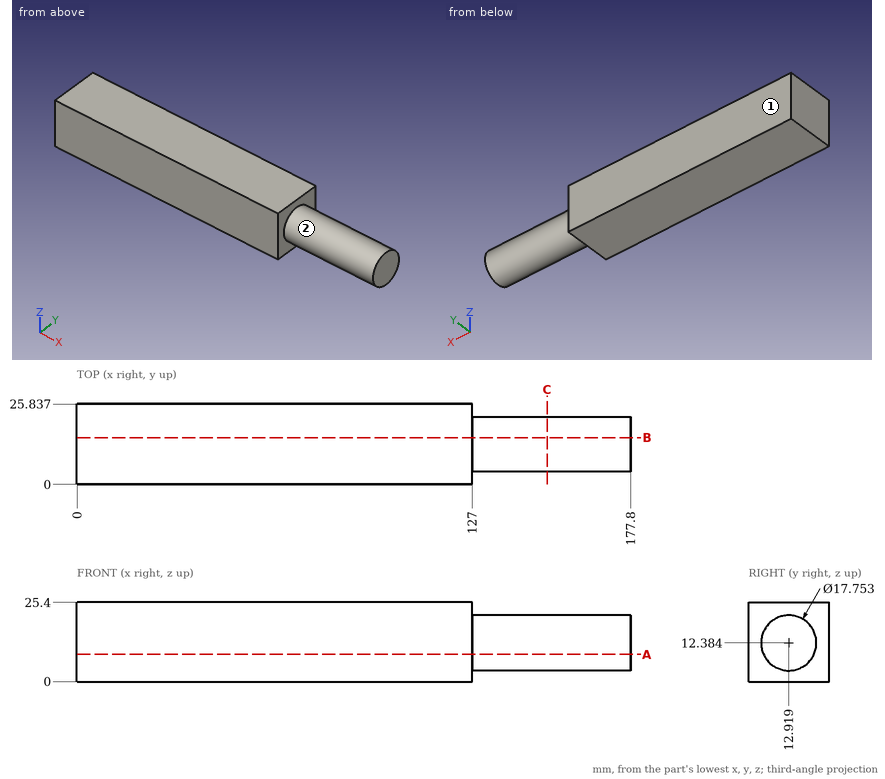
Here's the drawing with two shaded views (mm, measured from the low corner). I have some questions. A direction names the side the tool comes from. Coordinates: 2 decimals unless noted, no trailing zeros. Write each loop counter-clockwise with the first axis right and the second up, starting at its lowest first coordinate (ties: lowest second). Pieces come first, ordered by that corner, then holes. Notation, with made-up numbers: M 34.5,55 L 57.5,55 A6 ccw 57.5,66 Z; hole C 54.5,-13.75 d7. An arc over 180 degrees is marked long. Answer as CSV lines item,"result". Start each with the question number.
1) I want a section at A-A, the plane z = 8.75. Please give me the cut outline in (x, y), and give its area (3 significant figures).
2) I want a section at B-B, the plane y = 15. Please give me the cut outline in (x, z) (1 decimal).
3) For the marked faces 1 and 2, which set-ups out of +Z, -Z, +X, -X, +Y, -Y let a thin tool reach every point of the face, with its end or its side?
4) Please list where these lines run through material, in increasing order: line 1 (X direction, y = 5.5, z = 21.75); line 2 (Y direction, x = 142, z = 5) (1 decimal); line 3 (Z direction, x = 133, y = 19). Write a range as from..to.
5) I want a section at C-C, the plane x = 151. Please give me the cut outline in (y, z) (1 decimal).
6) For P1, Ø6, axis at x = 153.5, y = 7, coming from the -Z side, with a flat end and sliding along its axis, tell me the tip position at first contact or that it passes through.
Data:
1,outline,"M 0,0 L 127,0 L 127,4.82 L 177.8,4.82 L 177.8,21.02 L 127,21.02 L 127,25.84 L 0,25.84 Z"
1,area,"4,100 mm^2"
2,outline,"M 0,0 L 127,0 L 127,3.8 L 177.8,3.8 L 177.8,21 L 127,21 L 127,25.4 L 0,25.4 Z"
3,face 1,"+Z, -Z, +X, -X, +Y"
3,face 2,"+X"
4,line 1,"x = 0..127"
4,line 2,"y = 8..17.8"
4,line 3,"z = 5.92..18.85"
5,outline,"C 12.9,12.4 d17.8"
6,P1,"stops at z = 4"
